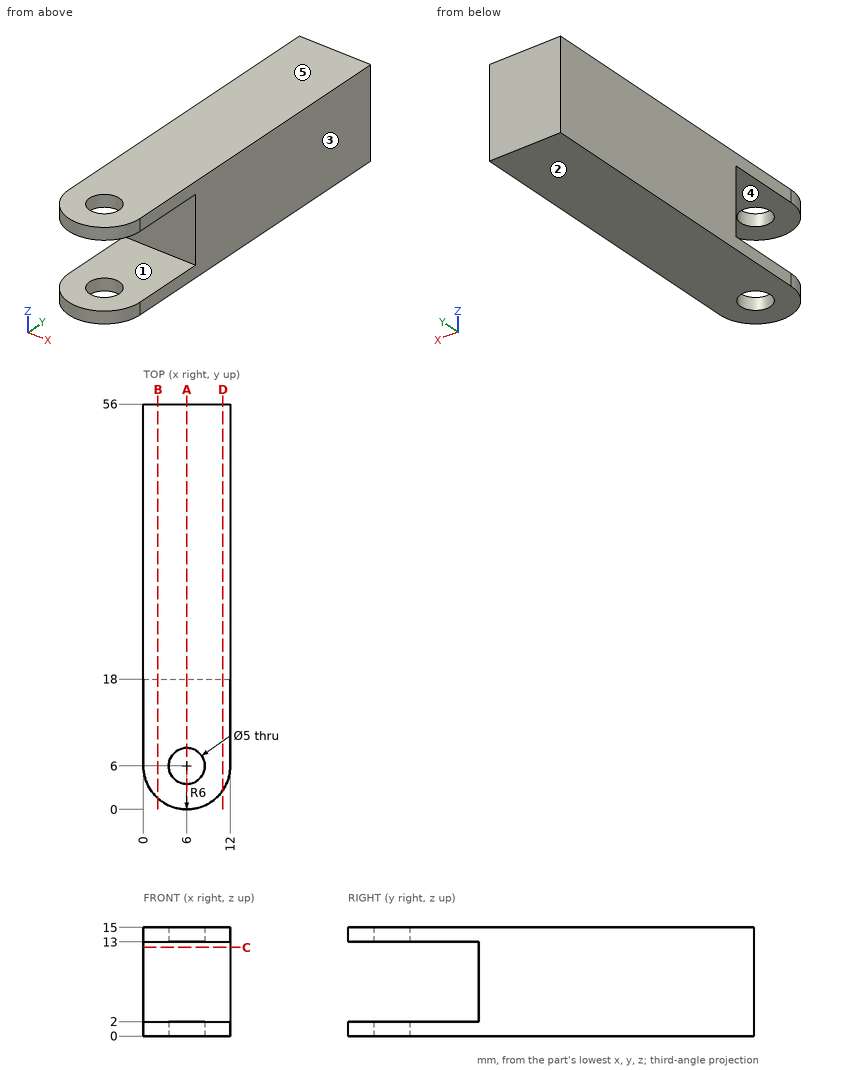
Job drawing, mm, ordinate dimensions from the low corner. One solid piece. A direction names the side the tool comes from. Coordinates: 2 decimals unless noted, no trailing zeros. Loops run counter-clockwise (first coordinate to the right, second up) from the corner with the lowest first, then second, coordinate; pieces in that order, holes last. Notation, with made-up numbers: (-33.75, 51.25) - (15.25, 51.25) arc R25 cw to (15.25, 64.25) - close; hole circle Ø6 at (-31.5, 27). An arc over 180 degrees is marked (long way). Answer as a JSON object with one key per item and string values. Group by question number.
(1) Cut at B-B (x = 2). Give the cut face in (y, z).
(2) Two-plate mould, pull along Z, no slides. Class the marked faces 3, 4 and 5: released by +Z, released by -Z, zero draft, split by the parting line, or undercut.
(3) Cut at A-A (x = 6). Give the cut face in (y, z), then the cut area to 3 significant figures.
(4) Tool access for the marked faces 1 and 2: list every direction of +Z, -Z, +X, -X, +Y, -Y with a clear straight run to the whole face (end or side of a thin tool).
(5) Cut at D-D (x = 11). Give the cut face in (y, z), then the cut area to 3 significant figures.
(6) Flat gauge pin, fed straight in: pin 1 (2 mm diameter, centred on x = 5, z = 10, fed in from -Y). Where does the tip first touch, or does it go through?
(7) Probe line 1 along X through (y, z) = (6, 14); line 2 along Y through (x, z) = (6, 14.6); line 3 along Z through (x, y) = (5, 17). List the from-to ranges inside material, lowest first.
(8) Cut at C-C (z = 12.25). Give the cut face in (x, y), then the cut area to 3 significant figures.
Geometry says:
{
 "1": {"outline": "(1.53, 0) - (56, 0) - (56, 15) - (1.53, 15) - (1.53, 13) - (18, 13) - (18, 2) - (1.53, 2) - close"},
 "2": {"face 3": "zero draft", "face 4": "undercut", "face 5": "released by +Z"},
 "3": {"outline": "(0, 0) - (3.5, 0) - (3.5, 2) - (0, 2) - close; (0, 13) - (3.5, 13) - (3.5, 15) - (0, 15) - close; (8.5, 0) - (56, 0) - (56, 15) - (8.5, 15) - (8.5, 13) - (18, 13) - (18, 2) - (8.5, 2) - close", "area": "622 mm^2"},
 "4": {"face 1": "+X, -X, -Y", "face 2": "-Z, +X, -X, +Y, -Y"},
 "5": {"outline": "(2.68, 0) - (56, 0) - (56, 15) - (2.68, 15) - (2.68, 13) - (18, 13) - (18, 2) - (2.68, 2) - close", "area": "631 mm^2"},
 "6": {"pin 1": "stops at y = 18"},
 "7": {"line 1": "x = 0 to 3.5, 8.5 to 12", "line 2": "y = 0 to 3.5, 8.5 to 56", "line 3": "z = 0 to 2, 13 to 15"},
 "8": {"outline": "(0, 18) - (12, 18) - (12, 56) - (0, 56) - close", "area": "456 mm^2"}
}
